Autodesk Inventor part; units mm, degrees
ref_plane "YZ Plane" through (0, 0, 0) normal (1, 0, 0) x (0, 1, 0)
ref_plane "XZ Plane" through (0, 0, 0) normal (0, 1, 0) x (-1, 0, 0)
ref_plane "XY Plane" through (0, 0, 0) normal (0, 0, 1) x (1, 0, 0)
sketch "Sketch1" plane through (0, 0, 0) normal (0, 1, 0) x (-1, 0, 0)
  circle A0 centre (0, 0) radius 14.5
  dimension "d0" = 29
extrude "Extrusion1" add sketch "Sketch1" along normal blind 3
sketch "Sketch2" plane through (0, 3, 0) normal (0, 1, 0) x (1, 0, 0)
  circle A0 centre (0, 0) radius 13.5
  dimension "d3" = 27
extrude "Extrusion2" cut sketch "Sketch2" against normal blind 0.5
sketch "Sketch3" plane through (0, 2.5, 0) normal (0, 1, 0) x (1, 0, 0)
  circle A0 centre (0, 0) radius 11
  circle A1 centre (0, 0) radius 5
  line L0 (-6.5333, 7.5044) -> (-3.8846, 4.462) construction
  line L1 (3.0432, 5.0733) -> (5.1182, 8.5325) construction
  arc A2 (4.6868, 9.9516) -> (-6.3569, 8.9771) centre (0, 0) ccw
  arc A3 (1.8214, 4.6564) -> (-2.6087, 4.2656) centre (0, 0) ccw
  line L2 (-7.2228, 8.2965) -> (-3.2831, 3.7711)
  line L3 (5.6584, 9.433) -> (2.572, 4.2877)
  arc A4 (-6.3569, 8.9771) -> (-6.5333, 7.5044) centre (-5.779, 8.161) ccw
  arc A5 (-3.8846, 4.462) -> (-2.6087, 4.2656) centre (-3.1304, 5.1187) ccw
  arc A6 (1.8214, 4.6564) -> (3.0432, 5.0733) centre (2.1857, 5.5877) ccw
  arc A7 (5.1182, 8.5325) -> (4.6868, 9.9516) centre (4.2607, 9.0469) ccw
  arc A8 (3.0991, 9.499) -> (-4.7146, 8.8096) centre (0.0131, -0.1481) ccw
  arc A9 (1.4786, 5.8357) -> (-2.4777, 5.4866) centre (-0.0344, 0.3898) ccw
  line L4 (-5.0021, 7.2686) -> (-3.6641, 5.7318)
  line L5 (3.652, 8.0321) -> (2.6039, 6.2848)
  arc A10 (-4.7146, 8.8096) -> (-5.0021, 7.2686) centre (-4.2478, 7.9252) ccw
  arc A11 (-3.6641, 5.7318) -> (-2.4777, 5.4866) centre (-2.9099, 6.3884) ccw
  arc A12 (1.4786, 5.8357) -> (2.6039, 6.2848) centre (1.7463, 6.7992) ccw
  arc A13 (3.652, 8.0321) -> (3.0991, 9.499) centre (2.7944, 8.5466) ccw
  arc A14 (9.9918, -0.0121) -> (6.9215, 7.2061) centre (-0.1369, -0.0582) ccw
  arc A15 (6.9215, 7.2061) -> (5.3671, 7.0033) centre (6.2246, 6.4889) ccw
  line L6 (5.3671, 7.0033) -> (4.319, 5.256)
  arc A16 (4.319, 5.256) -> (4.4525, 4.0519) centre (5.1765, 4.7416) ccw
  arc A17 (6.007, 0.3971) -> (4.4525, 4.0519) centre (0.3601, 0.1532) ccw
  arc A18 (6.007, 0.3971) -> (6.7819, -0.5343) centre (7.0061, 0.4402) ccw
  line L7 (8.7676, -0.9912) -> (6.7819, -0.5343)
  arc A19 (8.7676, -0.9912) -> (9.9918, -0.0121) centre (8.9918, -0.0166) ccw
  arc A20 (3.0761, -9.5065) -> (8.9923, -4.3559) centre (-0.0977, 0.1122) ccw
  arc A21 (8.9923, -4.3559) -> (8.3191, -2.9403) centre (8.0949, -3.9148) ccw
  line L8 (8.3191, -2.9403) -> (6.3334, -2.4834)
  arc A22 (6.3334, -2.4834) -> (5.2294, -2.9825) centre (6.1092, -3.4579) ccw
  arc A23 (2.2339, -5.5903) -> (5.2294, -2.9825) centre (0.2569, -0.2951) ccw
  arc A24 (2.2339, -5.5903) -> (1.5876, -6.615) centre (2.5837, -6.5271) ccw
  line L9 (1.7667, -8.6447) -> (1.5876, -6.615)
  arc A25 (1.7667, -8.6447) -> (3.0761, -9.5065) centre (2.7628, -8.5568) ccw
  arc A26 (-8.0906, -5.8632) -> (-1.3639, -9.8982) centre (0.0765, 0.1275) ccw
  arc A27 (-1.3639, -9.8982) -> (-0.2256, -8.8205) centre (-1.2217, -8.9084) ccw
  line L10 (-0.2256, -8.8205) -> (-0.4047, -6.7908)
  arc A28 (-0.4047, -6.7908) -> (-1.2205, -5.8951) centre (-1.4008, -6.8787) ccw
  arc A29 (-4.6264, -3.8521) -> (-1.2205, -5.8951) centre (-0.2013, -0.3355) ccw
  arc A30 (-4.6264, -3.8521) -> (-5.8007, -3.554) centre (-5.4093, -4.4742) ccw
  line L11 (-7.6757, -4.3516) -> (-5.8007, -3.554)
  arc A31 (-7.6757, -4.3516) -> (-8.0906, -5.8632) centre (-7.2843, -5.2718) ccw
  arc A32 (-8.0764, 5.8828) -> (-9.8353, -1.7615) centre (0.1449, -0.0333) ccw
  arc A33 (-9.8353, -1.7615) -> (-8.4585, -2.5111) centre (-8.8499, -1.5909) ccw
  line L12 (-8.4585, -2.5111) -> (-6.5835, -1.7136)
  arc A34 (-6.5835, -1.7136) -> (-5.9837, -0.6609) centre (-6.9749, -0.7934) ccw
  arc A35 (-5.0932, 3.2096) -> (-5.9837, -0.6609) centre (-0.3813, 0.0877) ccw
  arc A36 (-5.0932, 3.2096) -> (-5.1726, 4.4185) centre (-5.9268, 3.7619) ccw
  line L13 (-6.5105, 5.9553) -> (-5.1726, 4.4185)
  arc A37 (-6.5105, 5.9553) -> (-8.0764, 5.8828) centre (-7.2647, 5.2987) ccw
  point P0 (-10.1224, -4.3055)
  point P1 (0.9668, -10.9574)
  point P2 (10.7199, -2.4665)
  point P3 (-5.779, 8.161)
  point P4 (-3.1304, 5.1187)
  point P5 (2.1857, 5.5877)
  point P6 (3.9008, 4.5589)
  point P7 (5.9897, -0.352)
  point P8 (5.5412, -2.3011)
  point P9 (1.5161, -5.8053)
  point P10 (-0.4761, -5.9811)
  point P11 (-5.0527, -3.2358)
  point P12 (-5.8355, -1.3954)
  point P13 (-4.6388, 3.8054)
  dimension "d6" = 22
  dimension "d7" = 10
  dimension "d10" = 360
  dimension "d12" = 1
  dimension "d13" = 1
  dimension "d14" = 1
  dimension "d17" = 360
extrude "Extrusion3" cut sketch "Sketch3" against normal blind 0.4 contours A13 L5 A12 A9 A11 L4 A10 A8 | A19 L7 A18 A17 A16 L6 A15 A14 | A25 L9 A24 A23 A22 L8 A21 A20 | A31 L11 A30 A29 A28 L10 A27 A26 | A37 L13 A36 A35 A34 L12 A33 A32
sketch "Sketch4" plane through (0, 2.5, 0) normal (0, 1, 0) x (1, 0, 0)
  circle A0 centre (0, 0) radius 4
  dimension "d21" = 8
extrude "Extrusion4" add sketch "Sketch4" along normal blind 0.6
sketch "Sketch5" plane through (0, 3.1, 0) normal (0, 1, 0) x (1, 0, 0)
  circle A0 centre (0, 0) radius 2.5
  dimension "d24" = 5
extrude "Extrusion5" cut sketch "Sketch5" against normal blind 14.15
sketch "Sketch6" plane through (0, 0, 0) normal (0, -1, 0) x (1, 0, 0)
  circle A0 centre (0, 0) radius 2.5
  circle A1 centre (0, 0) radius 4.5
  dimension "d27" = 9
extrude "Extrusion6" add sketch "Sketch6" along normal blind 7.9
properties part number "inner_wheel" material "PAEK Plastic"
The model under review builds one solid part; all positions refer to its coordinate system, in mm. A direction names the side the tool comes from. Give positions to 0.01 mm unless a question says otherwise; leave off trailing zeros. Write each loop counter-clockwise with the first axis right and the second up, starting at its lowest first coordinate (ties: lowest second). Pieces come first, ordered by that corner, then holes.
(1) To check wall thickness, follow L1, parallel to Z at x = 0, y = 2.85; L2, parallel to Z at x = 0, y = -0.75; L3, parallel to Y at x = 9.25, z = -10. State the ranges of each line that lie inside material, in increasing order.
(2) Consider section C-C, the plane z = -11.75. Give the boundary of the cut face in (x, y), and give its area (3 significant figures).
(3) Tool access review of faces 3 (the cylindrical face through (-0.867, 2.796, -3.905)), 4 (the flat face through (2, 3.1, -2)): name each direction out of +Z, -Z, +X, -X, +Y, -Y from which nothing blocks a thin tool from reaching the whole face with its end or side.
(4) For P1, Ø1.5, axis at x = 8.5, z = 6.5, coming from the -Y side; P2, Ø3, axis at x = 6.5, z = -4.5, coming from the +Y side; P3, Ø5, axis at x = 1, z = -9, coming from the +Y side, all flat-tipped, find the tip position at first contact; note any pin that passes through.
(5) The part is to be moulded in two halves that separate along X. For faces 1 (the flat face through (-10, 3, -10)), 2 (the flat face through (-7, 2.1, -2)), say which applies: released by +X, released by -X, zero draft, split by the parting line, or undercut.
(6) Consider section D-D, the plane y = 0.75. Give the boundary of the cut face in (x, z).
(7) Consider section A-A, the plane y = -2. Give the boundary of the cut face in (x, z).
(8) Consider section B-B, the plane x = -7.25. Give the boundary of the cut face in (y, z).
Returned:
1. L1: z = -14.5 to -13.5, -4 to -2.5, 2.5 to 4, 13.5 to 14.5
1. L2: z = -4.5 to -2.5, 2.5 to 4.5
1. L3: y = 0 to 3
2. outline: (-8.5, 0) - (8.5, 0) - (8.5, 3) - (6.65, 3) - (6.65, 2.5) - (-6.65, 2.5) - (-6.65, 3) - (-8.5, 3) - close
2. area: 44.3 mm2
3. face 3: +Y
3. face 4: +Z, -Z, +X, -X, +Y
4. P1: stops at y = 0
4. P2: stops at y = 2.1
4. P3: stops at y = 2.5
5. face 1: zero draft
5. face 2: undercut
6. outline: circle Ø29 at (0, 0); hole circle Ø5 at (0, 0)
7. outline: circle Ø9 at (0, 0); hole circle Ø5 at (0, 0)
8. outline: (0, -12.56) - (3, -12.56) - (3, -11.39) - (2.5, -11.39) - (2.5, -6.3) - (2.1, -6.3) - (2.1, 2) - (2.5, 2) - (2.5, 4.17) - (2.1, 4.17) - (2.1, 6.87) - (2.5, 6.87) - (2.5, 11.39) - (3, 11.39) - (3, 12.56) - (0, 12.56) - close
